Answer from the drawing. Dimensions are ordinates in mm from the lowest x, y and z of the part. A direction names the side the tool comes from. Give positions to 0.01 mm unless a question says otherwise; leave off trailing zeros. Order: outer loops, then holes, each group sorted by start corner. A loop starts at its lowest first (then second) coordinate and runs counter-clockwise, first axis right, second up. Notation, with made-up numbers: (-31.5, -36) - (17.5, -36) arc R7 ccw to (17.5, -26) - close; hole circle Ø8 at (76, 83). An arc over 180 degrees is marked (long way). Write each question's results on one line, items separated by ' | '.
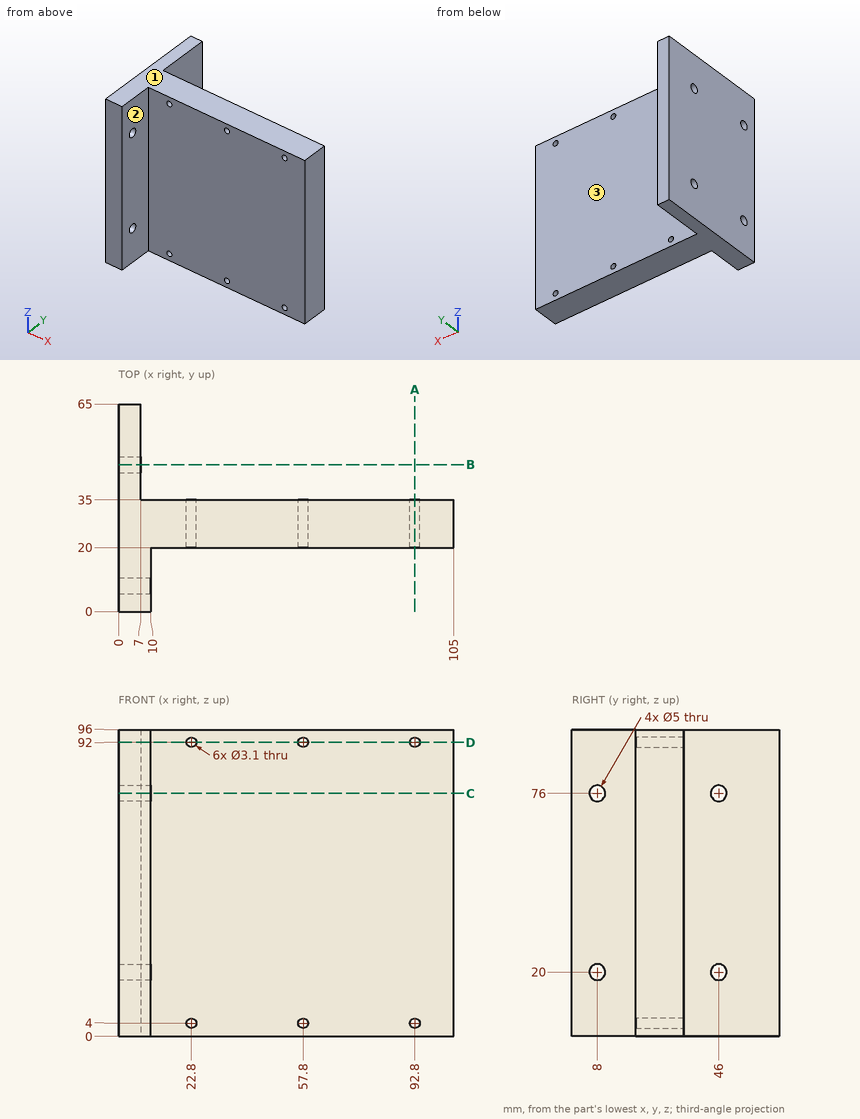
(1) Consider probe 1 along X at (y, z) = (31.25, 4); probe 2 along Y at (x, z) = (1.5, 76); probe 3 along Z at (x, y) = (22, 29). Determine where each line is inside the solid, lowest interval first. Write a range as [from, to].
Conclusion:
probe 1: [0, 21.25], [24.35, 56.25], [59.35, 91.25], [94.35, 105] | probe 2: [0, 5.5], [10.5, 43.5], [48.5, 65] | probe 3: [0, 2.67], [5.33, 90.67], [93.33, 96]
(2) Section A-A (x = 92.8) is taken. Give the vertices of the cut face in (y, z), plus the area to 3 significant figures.
Conclusion:
outline: (20, 0) - (35, 0) - (35, 2.45) - (20, 2.45) - close; (20, 5.55) - (35, 5.55) - (35, 90.45) - (20, 90.45) - close; (20, 93.55) - (35, 93.55) - (35, 96) - (20, 96) - close | area: 1,350 mm^2
(3) Each of these flat-tipped pins is pushed along its axis until it touches: pin 1 (4 mm diameter, centred on y = 8, z = 20, fed in from -X); pin 2 (4 mm diameter, centred on x = 92.8, z = 92, fed in from +Y); pin 3 (3 mm diameter, centred on y = 9.5, z = 14, fed in from +X); pin 4 (10 mm diameter, centred on x = 71.5, z = 26, fed in from -Y). Where does it stop, or does it pass through?
Conclusion:
pin 1: through | pin 2: y = 35 | pin 3: x = 10 | pin 4: y = 20
(4) For the marked faces 1, 2 and 3, determine the directions among +Z, -Z, +X, -X, +Y, -Y from which every point of the face is accessible in a straight line to the end or side of a thin tool.
Conclusion:
face 1: +Z, +X, -X, +Y, -Y | face 2: +Z, -Z, +X, -Y | face 3: +Z, -Z, +X, +Y
(5) Section C-C (z = 76) is taken. Give the vertices of the cut face in (x, y).
Conclusion:
outline: (0, 0) - (10, 0) - (10, 5.5) - (0, 5.5) - close; (0, 10.5) - (10, 10.5) - (10, 20) - (105, 20) - (105, 35) - (7, 35) - (7, 43.5) - (0, 43.5) - close; (0, 48.5) - (7, 48.5) - (7, 65) - (0, 65) - close
(6) Section B-B (y = 46) is taken. Give the vertices of the cut face in (x, z), plus the area to 3 significant figures.
Conclusion:
outline: (0, 0) - (7, 0) - (7, 17.5) - (0, 17.5) - close; (0, 22.5) - (7, 22.5) - (7, 73.5) - (0, 73.5) - close; (0, 78.5) - (7, 78.5) - (7, 96) - (0, 96) - close | area: 602 mm^2
(7) Section D-D (z = 92) is taken. Give the vertices of the cut face in (x, y), plus the area to 3 significant figures.
Conclusion:
outline: (0, 0) - (10, 0) - (10, 20) - (21.25, 20) - (21.25, 35) - (7, 35) - (7, 65) - (0, 65) - close; (24.35, 20) - (56.25, 20) - (56.25, 35) - (24.35, 35) - close; (59.35, 20) - (91.25, 20) - (91.25, 35) - (59.35, 35) - close; (94.35, 20) - (105, 20) - (105, 35) - (94.35, 35) - close | area: 1,850 mm^2
